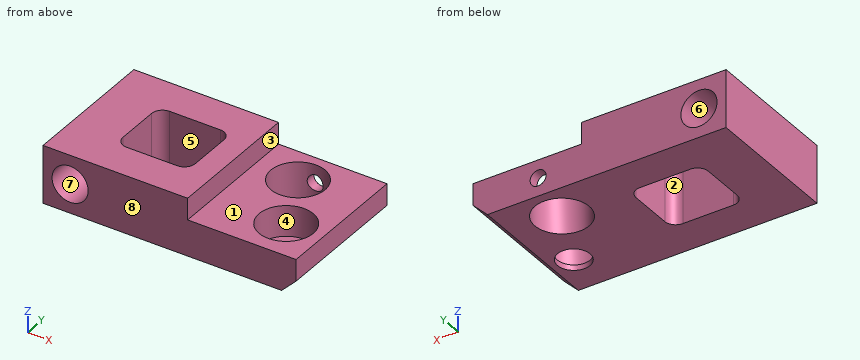
```python
from build123d import *

# Parameters (mm, degrees)
F0_W            = 70
F0_H            = 38
F1_DEPTH        = 16
F3_D            = 9
F3_DEPTH        = 28
F3_CBORE_D      = 10
F3_CBORE_DEPTH  = 10
F3_TIP          = 2.7038727856
F5_D            = 9
F5_DEPTH        = 28
F5_CBORE_D      = 10
F5_CBORE_DEPTH  = 10
F5_TIP          = 2.7038727856
F7_DEPTH        = 25
F8_W            = 30
F8_H            = 38
F9_DEPTH        = 6
F10_SIZE        = 4
F12_D           = 9
F12_DEPTH       = 28
F12_CBORE_D     = 15
F12_CBORE_DEPTH = 8.5
F12_TIP         = 2.7038727856
F14_D           = 15
F14_DEPTH       = 28
F14_TIP         = 4.5064546427
F16_D           = 4.4
F16_DEPTH       = 10
F16_TIP         = 1.3218933619


with BuildPart() as f1:
    # F0 (on Top) → F1 (new body)
    with BuildSketch(Plane.XY):
        Rectangle(F0_W, F0_H)
    extrude(amount=F1_DEPTH)

    # F3
    with Locations(Plane.XZ.offset(19)):
        with Locations((-27.5, 8)):
            CounterBoreHole(F3_D / 2, F3_CBORE_D / 2, F3_CBORE_DEPTH, depth=F3_DEPTH)
            with Locations((0, 0, -(F3_DEPTH + F3_TIP / 2))):  # 118° drill point
                Cone(0, F3_D / 2, F3_TIP, mode=Mode.SUBTRACT)

    # F5
    with Locations(Plane(origin=(0, 19, 0), x_dir=(-1, 0, 0), z_dir=(0, 1, 0))):
        with Locations((27.5, 8)):
            CounterBoreHole(F5_D / 2, F5_CBORE_D / 2, F5_CBORE_DEPTH, depth=F5_DEPTH)
            with Locations((0, 0, -(F5_DEPTH + F5_TIP / 2))):  # 118° drill point
                Cone(0, F5_D / 2, F5_TIP, mode=Mode.SUBTRACT)

    # F6 (on face) → F7 (cut)
    with BuildSketch(Plane.XY.offset(16)):
        with BuildLine():
            Line((-4.5, 9), (-18.5, 9))
            ThreePointArc((-18.5, 9), (-20.6213203436, 8.1213203436), (-21.5, 6))
            Line((-21.5, 6), (-21.5, -6))
            ThreePointArc((-21.5, -6), (-20.6213203436, -8.1213203436), (-18.5, -9))
            Line((-18.5, -9), (-4.5, -9))
            ThreePointArc((-4.5, -9), (-2.3786796564, -8.1213203436), (-1.5, -6))
            Line((-1.5, -6), (-1.5, 6))
            ThreePointArc((-1.5, 6), (-2.3786796564, 8.1213203436), (-4.5, 9))
        make_face()
    extrude(amount=-F7_DEPTH, mode=Mode.SUBTRACT)

    # F8 (on face) → F9 (cut)
    with BuildSketch(Plane.XY.offset(16)):
        with Locations((20, 0)):
            Rectangle(F8_W, F8_H)
    extrude(amount=-F9_DEPTH, mode=Mode.SUBTRACT)

    # F10
    f10_edges = [f1.edges().sort_by_distance(p)[0] for p in [
        (35, 0, 0),
    ]]
    chamfer(f10_edges, length=F10_SIZE)

    # F12
    with Locations(Plane.XY.offset(10)):
        with Locations((24.789, -7.6924054883)):
            CounterBoreHole(F12_D / 2, F12_CBORE_D / 2, F12_CBORE_DEPTH, depth=F12_DEPTH)
            with Locations((0, 0, -(F12_DEPTH + F12_TIP / 2))):  # 118° drill point
                Cone(0, F12_D / 2, F12_TIP, mode=Mode.SUBTRACT)

    # F14
    with Locations(Plane.XY.offset(10)):
        with Locations((17, 9)):
            Hole(F14_D / 2, depth=F14_DEPTH)
            with Locations((0, 0, -(F14_DEPTH + F14_TIP / 2))):  # 118° drill point
                Cone(0, F14_D / 2, F14_TIP, mode=Mode.SUBTRACT)

    # F16
    with Locations(Plane(origin=(0, 19, 0), x_dir=(-1, 0, 0), z_dir=(0, 1, 0))):
        with Locations((-17, 5)):
            Hole(F16_D / 2, depth=F16_DEPTH)
            with Locations((0, 0, -(F16_DEPTH + F16_TIP / 2))):  # 118° drill point
                Cone(0, F16_D / 2, F16_TIP, mode=Mode.SUBTRACT)


solid = f1.part
```
Source: CAD feature listing. Evaluate the final solid. Frame: model axes, mm. Face numbers are marked on the shaded views. A direction names the side the tool comes from. Give positions to 0.01 mm unless a question says otherwise; leave off trailing zeros. Order: outer loops, then holes, each group sorted by start corner. A loop starts at its lowest first (then second) coordinate and runs counter-clockwise, first axis right, second up. Notation, with made-up numbers: (1.25, 48.5) -> (58.25, 48.5) arc R19 ccw to (58.25, 71.5) -> close; hole circle Ø5 at (88, -13.5). An arc over 180 degrees is marked (long way). Use a Markdown table: item, result.
Q1. Pull-direction query (X, two-part tool) for the marked faces 1, 2 and 3; classes: +X half, -X half, draft (parallel to the pull), parting line (faces both ways), or undercut.
A:
| item | result |
|---|---|
| face 1 | draft |
| face 2 | undercut |
| face 3 | +X half |
Q2. Material intervals for line 1 (X direction, y = 0.25, z = 8); line 2 (X direction, y = -2, z = 8.75); line 3 (X direction, y = 7, z = 4.5), sorted ascending. Write a range as [from, to].
A:
| item | result |
|---|---|
| line 1 | [-35, -32], [-23, -21.5], [-1.5, 35] |
| line 2 | [-35, -31.94], [-23.06, -21.5], [-1.5, 19.91], [29.67, 35] |
| line 3 | [-35, -30.33], [-24.67, -21.33], [-1.67, 9.77], [24.23, 35] |
Q3. First-contact query: P1, Ø15, axis at x = 18, y = 8, coming from the +Z side; P2, Ø7, axis at x = -27.5, z = 8, coming from the +Y side; P3, Ø10.5, axis at x = 24.79, y = -7.69, coming from the +Z side; P4, Ø1.8, axis at y = -8, z = 11.5, coming from the +X side. Flat tips, straight axial feed; report the tip coordinate or a pass-through.
A:
| item | result |
|---|---|
| P1 | z = 10 |
| P2 | through |
| P3 | z = 1.5 |
| P4 | x = 5 |
Q4. Section C-C (x = -27.5). Return the cut outline in (y, z).
A:
| item | result |
|---|---|
| outline | (-19, 0) -> (19, 0) -> (19, 3) -> (9, 3) -> (9, 3.5) -> (-9, 3.5) -> (-9, 3) -> (-19, 3) -> close; (-19, 13) -> (-9, 13) -> (-9, 12.5) -> (9, 12.5) -> (9, 13) -> (19, 13) -> (19, 16) -> (-19, 16) -> close |
Q5. Section D-D (z = 8). Return the cut outline in (x, y), and give its area (3 significant figures).
A:
| item | result |
|---|---|
| outline | (-35, -19) -> (-32.5, -19) -> (-32.5, -9) -> (-32, -9) -> (-32, 9) -> (-32.5, 9) -> (-32.5, 19) -> (-35, 19) -> close; (-23, -9) -> (-22.5, -9) -> (-22.5, -19) -> (35, -19) -> (35, 19) -> (-22.5, 19) -> (-22.5, 9) -> (-23, 9) -> close; hole (-21.5, -6) arc R3 ccw to (-18.5, -9) -> (-4.5, -9) arc R3 ccw to (-1.5, -6) -> (-1.5, 6) arc R3 ccw to (-4.5, 9) -> (-18.5, 9) arc R3 ccw to (-21.5, 6) -> close; hole circle Ø15 at (17, 9); hole circle Ø15 at (24.79, -7.69) |
| area | 1,590 mm^2 |
Q6. Section A-A (z = 5). State how many separate pieces and enclosed holes the cut face has, and give its area (3 significant figures).
A:
| item | result |
|---|---|
| separate pieces | 2 |
| enclosed holes | 2 |
| area | 1,660 mm^2 |
Q7. Access query for the marked faces 4, 5, 6, 7 and 8. Directions: +Z, -Z, +X, -X, +Y, -Y. A direction counts if a zero-diameter tool reaches every point of the face in a straight line with its end or side. Return the directions, or none.
A:
| item | result |
|---|---|
| face 4 | +Z |
| face 5 | +Z, -Z |
| face 6 | +Y |
| face 7 | -Y |
| face 8 | +Z, -Z, +X, -X, -Y |
Q8. Section B-B (y = -1). Return the cut outline in (x, z), and give its area (3 significant figures).
A:
| item | result |
|---|---|
| outline | (-35, 0) -> (-21.5, 0) -> (-21.5, 16) -> (-35, 16) -> close; (-1.5, 0) -> (31, 0) -> (35, 4) -> (35, 10) -> (28.17, 10) -> (28.17, 1.5) -> (21.4, 1.5) -> (21.4, 10) -> (5, 10) -> (5, 16) -> (-1.5, 16) -> close; hole circle Ø9 at (-27.5, 8) |
| area | 491 mm^2 |
